```python
from build123d import *

# Parameters (mm, degrees)
F0_R     = 10.93658
F1_DEPTH = 76.2
F2_DEPTH = 101.6


with BuildPart() as f1:
    # F0 (on Right) → F1 (new body, symmetric)
    with BuildSketch(Plane.YZ):
        Polygon((-12.313237, -10.17919), (-20.806385, -32.049883), (20.806385, -32.049883), (12.313237, -10.17919), align=None)
        with BuildLine():
            ThreePointArc((-29.184296, 9.448227), (-85.59756, 19.031296), (-59.809873, -32.049883))
            Line((-59.809873, -32.049883), (-20.806385, -32.049883))
            Line((-20.806385, -32.049883), (-12.313237, -10.17919))
            Line((-12.313237, -10.17919), (-9.436439, 9.448227))
            Line((-9.436439, 9.448227), (-29.184296, 9.448227))
        make_face()
        with Locations((-59.809873, 0)):
            Circle(F0_R, mode=Mode.SUBTRACT)
        Polygon((-9.436439, 9.448227), (-12.313237, -10.17919), (12.313237, -10.17919), (9.436439, 9.448227), align=None)
        with BuildLine():
            Line((12.313237, -10.17919), (20.806385, -32.049883))
            Line((20.806385, -32.049883), (59.809873, -32.049883))
            ThreePointArc((59.809873, -32.049883), (85.59756, 19.031296), (29.184296, 9.448227))
            Line((29.184296, 9.448227), (9.436439, 9.448227))
            Line((9.436439, 9.448227), (12.313237, -10.17919))
        make_face()
        with Locations((59.809873, 0)):
            Circle(F0_R, mode=Mode.SUBTRACT)
    extrude(amount=F1_DEPTH, both=True)

    # F0 (on Right) → F2 (join, symmetric)
    with BuildSketch(Plane.YZ):
        Polygon((-12.313237, -10.17919), (-20.806385, -32.049883), (20.806385, -32.049883), (12.313237, -10.17919), align=None)
        Polygon((-9.436439, 9.448227), (-12.313237, -10.17919), (12.313237, -10.17919), (9.436439, 9.448227), align=None)
    extrude(amount=F2_DEPTH, both=True)


solid = f1.part
```
Read the model definition and answer for the solid it produces. Units are mm, in the model's axes. A direction names the side the tool comes from. Coordinates: 2 decimals unless noted, no trailing zeros. Write each loop counter-clockwise with the first axis right and the second up, starting at its lowest first coordinate (ties: lowest second). Pieces come first, ordered by that corner, then holes. Notation, with made-up numbers: (-23, 38) - (16, 38) arc R26 cw to (16, 68) - close; hole circle Ø6 at (60.5, -11.75). An arc over 180 degrees is marked (long way). Answer as a JSON object with one key per item and string values. Group by question number.
1. A cutting plane is placed at C-C (x = -43). Determine the outline of the cut face in (y, z).
2. The mould has two halves that part along Y. Classify faces 6 (the flat face through (89.078, -10.855, -0.228)), 7 (the cylindrical face through (1.07, 86.17, 18.23)), 8 (the flat face through (76.2, 50, -7)): +Y half, -Y half, draft (parallel to the pull), parting line (faces both ways), or undercut.
3. Each of these flat-tipped pins is pushed along its axis until it touches: P1, Ø1, axis at y = 68, z = 13.5, coming from the +X side; P2, Ø1, axis at x = 31.5, z = 9, coming from the -Y side; P3, Ø2, axis at y = -54, z = -23, coming from the -X side. Where does it stop, or does it pass through?
4. A cutting plane is placed at B-B (y = 66). Determine the outline of the cut face in (x, z), plus the area to 3 significant figures.
5. Which of the six approach directions +Z, -Z, +X, -X, +Y, -Y give full straight-line access (tool end or side, diameter ignored) to faces 1 (the flat face through (89.08, -16.5, -20.96)), 2 (the flat face through (89.078, 10.895, -0.503)), 3 (the flat face through (-88.72, 16.62, -21.27)), 4 (the flat face through (-88.722, -10.855, -0.228)), 5 (the flat face through (1, 0, 9.448))?
6. A cutting plane is placed at A-A (z = 0). Determine the outline of the cut face in (x, y), plus the area to 3 significant figures.
7. A cutting plane is placed at D-D (z = 22). Determine the outline of the cut face in (x, y).
8. Consider L1, parallel to Y at x = -59.5, z = -10; L2, parallel to Y at x = -56, z = -9.5; L3, parallel to Z at x = 55, y = -23. Determine where each line is inside the solid, lowest interval first. Write a range as [from, to].
Worked out:
{
 "1": {"outline": "(-59.81, -32.05) - (59.81, -32.05) arc R32.05 ccw (long way) to (29.18, 9.45) - (-29.18, 9.45) arc R32.05 ccw (long way) to start; hole circle Ø21.87 at (-59.81, 0); hole circle Ø21.87 at (59.81, 0)"},
 "2": {"face 6": "-Y half", "face 7": "undercut", "face 8": "draft"},
 "3": {"P1": "stops at x = 76.2", "P2": "stops at y = -90.71", "P3": "stops at x = -76.2"},
 "4": {"outline": "(-76.2, -31.45) - (76.2, -31.45) - (76.2, -9.02) - (-76.2, -9.02) - close; (-76.2, 9.02) - (76.2, 9.02) - (76.2, 31.45) - (-76.2, 31.45) - close", "area": "6,840 mm²"},
 "5": {"face 1": "+Z, +X, -Y", "face 2": "+Z, +X, +Y", "face 3": "+Z, -X, +Y", "face 4": "+Z, -X, -Y", "face 5": "+Z, +X, -X"},
 "6": {"outline": "(-101.6, -10.82) - (-76.2, -10.82) - (-76.2, -48.87) - (76.2, -48.87) - (76.2, -10.82) - (101.6, -10.82) - (101.6, 10.82) - (76.2, 10.82) - (76.2, 48.87) - (-76.2, 48.87) - (-76.2, 10.82) - (-101.6, 10.82) - close; (-76.2, -91.86) - (76.2, -91.86) - (76.2, -70.75) - (-76.2, -70.75) - close; (-76.2, 70.75) - (76.2, 70.75) - (76.2, 91.86) - (-76.2, 91.86) - close", "area": "22,400 mm²"},
 "7": {"outline": "(-76.2, -83.12) - (76.2, -83.12) - (76.2, -36.5) - (-76.2, -36.5) - close; (-76.2, 36.5) - (76.2, 36.5) - (76.2, 83.12) - (-76.2, 83.12) - close"},
 "8": {"L1": "y = [-90.26, -64.24], [-55.38, 55.38], [64.24, 90.26]", "L2": "y = [-90.42, -65.23], [-54.39, 54.39], [65.23, 90.42]", "L3": "z = [-32.05, 9.45]"}
}
